Input: part model. Units: mm. Frame: model coordinates. A direction names the side the tool comes from. Round coordinates to 2 decimals unless told otherwise and drop trailing zeros. Loops run counter-clockwise (first coordinate to the right, second up) from the corner with the lowest first, then second, coordinate; pieces in that order, holes last. Notation, with made-up numbers: (52.25, -17) -> (110.25, -17) arc R23 cw to (110.25, -1) -> close; hole circle Ø1 at (40.5, 76). An arc over 180 degrees is marked (long way). One line per question, with ' | ' between items. Start each with the question number.
Q1. Access query for faces 4 (the face through (-5.5, 0, 2)), 5 (the face through (1, 0, 3.4)), 6 (the face through (-4.232, -0.065, 1.504)), 7 (the face through (-1, 0, 3.4)). Directions: +Z, -Z, +X, -X, +Y, -Y. A direction counts if a zero-diameter tool reaches every point of the face in a straight line with its end or side. Return the directions, or none.
Q2. Mould query, pull axis X, two halves, no side actions, for faces 1 (the face through (-1, 0, 0.5)), 2 (the face through (0.525, 0.165, 1.972)), 3 (the face through (4.232, -0.065, 1.504)). Classes: pulls with the +X half, pulls with the -X half, needs draft (parallel to the pull), parting line crosses it, or undercut.
Q3. Contact query for flat-ended pins moving along their axis: P1, Ø1, axis at x = 2.5, z = 3, coming from the +Y side; P2, Ø1, axis at x = 2, y = -0.5, coming from the +Z side; P3, Ø0.6, axis at y = 0, z = 3.5, coming from the +X side. Output: stop coordinate, or through.
Q4. Material intervals for L1, parallel to Y at x = 0, z = 1.9; L2, parallel to Z at x = 3, y = 0.05; L3, parallel to Y at x = -3.5, z = 2.4, sorted ascending.
Q5. Cut plane B-B on x = 0. Return loops of the section in (y, z).
Q6. Cut plane C-C on z = 3.7. Return loops of the section in (x, y), and give its area (3 significant figures).
Q7. Cut plane D-D on x = 4. Return loops of the section in (y, z).
Q8. Cut plane A-A on y = 0. Return loops of the section in (x, z).
from build123d import *

# Parameters (mm, degrees)
SKETCH1_W           = 2
SKETCH1_H           = 2
SKETCH1_R           = 0.55
BOSS_EXTRUDE1_DEPTH = 4


with BuildPart() as part:
    # Sketch1 → Boss-Extrude1 (new body)
    with BuildSketch(Plane.XY):
        Rectangle(SKETCH1_W, SKETCH1_H)
        Circle(SKETCH1_R, mode=Mode.SUBTRACT)
    extrude(amount=BOSS_EXTRUDE1_DEPTH)

    # 草图1 → 旋转1 (revolve)
    with BuildSketch(Plane.XY.offset(2)):
        Polygon((1, 1), (1, 0), (5.5, 0), (5.5, 0.5), (3, 0.5), align=None)
        Polygon((-1, 0), (-5.5, 0), (-5.5, 0.5), (-3, 0.5), (-1, 1), align=None)
    revolve(axis=Axis((-1, 0, 2), (-1, 0, 0)))


solid = part.part
Results:
1) face 4: +Z, -Z, -X, +Y, -Y | face 5: +Z, +X | face 6: -X | face 7: +Z, -X
2) face 1: pulls with the -X half | face 2: undercut | face 3: needs draft
3) P1: y = 0.41 | P2: z = 2.83 | P3: x = 1
4) L1: -1 to -0.55, 0.55 to 1 | L2: 1.5 to 2.5 | L3: -0.3 to 0.3
5) outline: (-1, 0) -> (-0.55, 0) -> (-0.55, 4) -> (-1, 4) -> close; (0.55, 0) -> (1, 0) -> (1, 4) -> (0.55, 4) -> close
6) outline: (-1, -1) -> (1, -1) -> (1, 1) -> (-1, 1) -> close; hole circle Ø1.1 at (0, 0) | area: 3.05 mm^2
7) outline: circle Ø1 at (0, 2)
8) outline: (-5.5, 1.5) -> (-3, 1.5) -> (-1, 1) -> (-1, 0) -> (-0.55, 0) -> (-0.55, 4) -> (-1, 4) -> (-1, 3) -> (-3, 2.5) -> (-5.5, 2.5) -> close; (0.55, 0) -> (1, 0) -> (1, 1) -> (3, 1.5) -> (5.5, 1.5) -> (5.5, 2.5) -> (3, 2.5) -> (1, 3) -> (1, 4) -> (0.55, 4) -> close
